Here's how the part is built. I have some questions about the finished solid (model axes, mm). Face numbers are marked on the shaded views. A direction names the side the tool comes from. Give positions to 0.01 mm unless a question says otherwise; leave off trailing zeros. Order: outer loops, then holes, each group sorted by start corner. A loop starts at its lowest first (then second) coordinate and runs counter-clockwise, first axis right, second up.
from build123d import *

# Parameters (mm, degrees)
SKETCH_1_W          = 40
SKETCH_1_H          = 50
EXTRUDE_1_DEPTH     = 8
SKETCH_2_W          = 40
SKETCH_2_H          = 8
EXTRUDE_2_DEPTH     = 70
SKETCH_3_R          = 3.25
CUT_EXTRUDE_1_DEPTH = 9
SKETCH_4_R          = 3.25
CUT_EXTRUDE_2_DEPTH = 8


with BuildPart() as part:
    # 草图1 → 凸台-拉伸1 (new body)
    with BuildSketch(Plane.XY):
        with Locations((0, -25)):
            Rectangle(SKETCH_1_W, SKETCH_1_H)
    extrude(amount=EXTRUDE_1_DEPTH)

    # 草图2 → 凸台-拉伸2 (add)
    with BuildSketch(Plane.XY):
        with Locations((0, -4)):
            Rectangle(SKETCH_2_W, SKETCH_2_H)
    extrude(amount=EXTRUDE_2_DEPTH)

    # 草图3 → 切除-拉伸1 (cut)
    with BuildSketch(Plane(origin=(0, 0, 0), x_dir=(-1, 0, 0), z_dir=(0, 0, -1))):
        with Locations((0, -20)):
            Circle(SKETCH_3_R)
        with Locations((0, -40)):
            Circle(SKETCH_3_R)
    extrude(amount=-CUT_EXTRUDE_1_DEPTH, mode=Mode.SUBTRACT)

    # 草图4 → 切除-拉伸2 (cut)
    with BuildSketch(Plane.XZ.offset(8)):
        with Locations(Location((0, 34, 0), (0, 0, 270))):
            Circle(SKETCH_4_R)
        with Locations(Location((0, 54, 0), (0, 0, 270))):
            Circle(SKETCH_4_R)
    extrude(amount=-CUT_EXTRUDE_2_DEPTH, mode=Mode.SUBTRACT)


solid = part.part
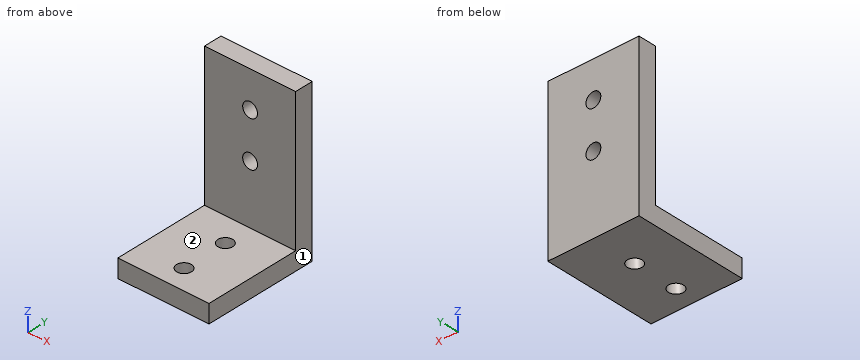
Q1. If we section it at C-C on x = 0: List the corners of the cut face in (y, z) for me, plus the area to 3 significant figures.
Filled sheet:
outline: (-50, 0) - (-43.25, 0) - (-43.25, 8) - (-50, 8) - close; (-36.75, 0) - (-23.25, 0) - (-23.25, 8) - (-36.75, 8) - close; (-16.75, 0) - (0, 0) - (0, 30.75) - (-8, 30.75) - (-8, 8) - (-16.75, 8) - close; (-8, 37.25) - (0, 37.25) - (0, 50.75) - (-8, 50.75) - close; (-8, 57.25) - (0, 57.25) - (0, 70) - (-8, 70) - close
area: 688 mm2
Q2. I need wall thicknesses on L1, parallel to Y at x = 0, z = 2.75; L2, parallel to X at y = -4, z = 34; L3, parallel to Y at x = 18, z = 58. Which ranges of each line are inside material? Lowest first, please.
Filled sheet:
L1: y = -50 to -43.25, -36.75 to -23.25, -16.75 to 0
L2: x = -20 to -3.25, 3.25 to 20
L3: y = -8 to 0
Q3. For the marked faces 1 and 2, which set-ups out of +Z, -Z, +X, -X, +Y, -Y let a thin tool reach every point of the face, with its end or its side?
Filled sheet:
face 1: +Z, -Z, +X, +Y, -Y
face 2: +Z, +X, -X, -Y
Q4. I'm going to push flat-ended pins straight in: P1, Ø7.5, axis at x = 0, z = 54, coming from the -Y side; P2, Ø4, axis at x = 0, y = -20, coming from the +Z side; P3, Ø12, axis at x = -5, y = -39.5, coming from the +Z side. Where does each tip first touch, or does it pass through?
Filled sheet:
P1: stops at y = -8
P2: passes through
P3: stops at z = 8
Q5. If we section it at A-A on z = 54: List the corners of the cut face in (x, y) for me.
Filled sheet:
outline: (-20, -8) - (-3.25, -8) - (-3.25, 0) - (-20, 0) - close; (3.25, -8) - (20, -8) - (20, 0) - (3.25, 0) - close
Q6. If we section it at B-B on y = -40: List the corners of the cut face in (x, z) for me, plus the area to 3 significant figures.
Filled sheet:
outline: (-20, 0) - (-3.25, 0) - (-3.25, 8) - (-20, 8) - close; (3.25, 0) - (20, 0) - (20, 8) - (3.25, 8) - close
area: 268 mm2
Q7. If we section it at D-D on y = -7: List the corners of the cut face in (x, z) for me.
Filled sheet:
outline: (-20, 0) - (20, 0) - (20, 70) - (-20, 70) - close; hole circle Ø6.5 at (0, 34); hole circle Ø6.5 at (0, 54)
